Here's the drawing with two shaded views (mm, measured from the low corner). I have some questions. A direction names the side the tool comes from. Coordinates: 2 decimals unless noted, no trailing zeros. Loops run counter-clockwise (first coordinate to the right, second up) from the corner with the lowest first, then second, coordinate; pieces in that order, holes last. Notation, with made-up numbers: (62, -7) - (115, -7) arc R21 ccw to (115, 27) - close; hole circle Ø1 at (-33.5, 47). An arc over 180 degrees is marked (long way). Use a Markdown table: item, result.
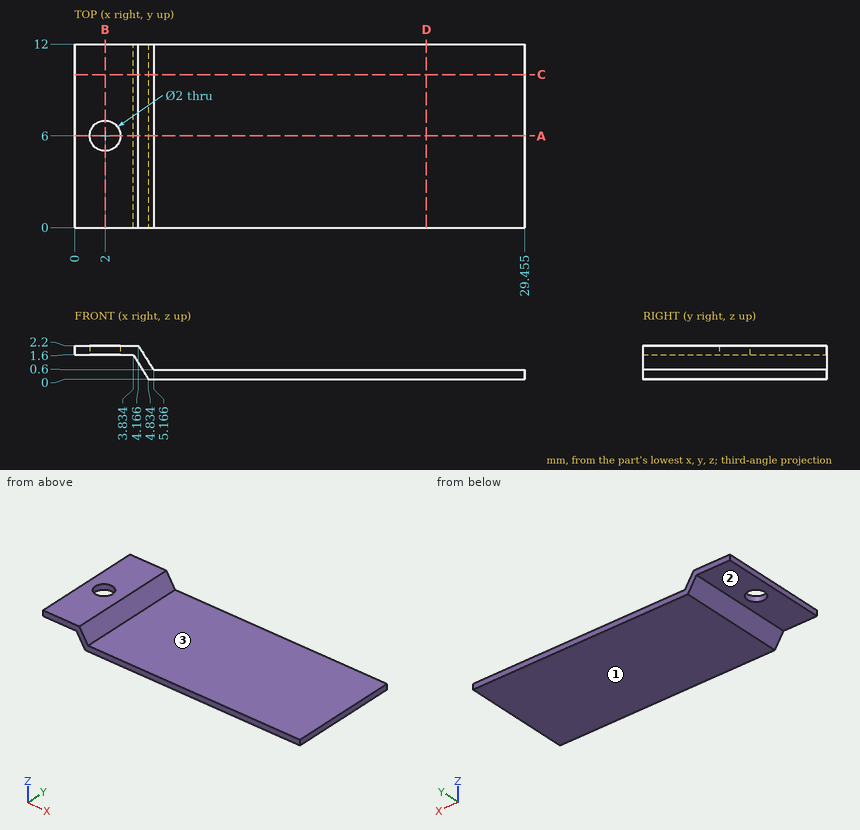
Q1. I want a section at D-D, the plane x = 23. Write out the boundary of the cut face in (y, z).
Check values:
| item | result |
|---|---|
| outline | (0, 0) - (12, 0) - (12, 0.6) - (0, 0.6) - close |
Q2. I want a section at A-A, the plane y = 6. Write out the boundary of the cut face in (x, z) (1 decimal), then the cut area to 3 significant figures.
Check values:
| item | result |
|---|---|
| outline | (0, 1.6) - (1, 1.6) - (1, 2.2) - (0, 2.2) - close; (3, 1.6) - (3.8, 1.6) - (4.8, 0) - (29.5, 0) - (29.5, 0.6) - (5.2, 0.6) - (4.2, 2.2) - (3, 2.2) - close |
| area | 17.0 mm^2 |
Q3. Please list where these lines run through material, in increasing order: L1, parallel to Z at x = 24.5, y = 4.5; L2, parallel to X at y = 6, z = 2.1; L3, parallel to X at y = 5.5, z = 1.7 (1 decimal). Write a range as from..to.
Check values:
| item | result |
|---|---|
| L1 | 0..0.6 |
| L2 | 0..1, 3..4.23 |
| L3 | 0..1.1, 2.9..4.5 |
Q4. I want a section at B-B, the plane x = 2. Write out the boundary of the cut face in (y, z).
Check values:
| item | result |
|---|---|
| outline | (0, 1.6) - (5, 1.6) - (5, 2.2) - (0, 2.2) - close; (7, 1.6) - (12, 1.6) - (12, 2.2) - (7, 2.2) - close |
Q5. Which directions (+Z, -Z, +X, -X, +Y, -Y) give clear straight access to the entire face, cutting with the end or side of a thin tool? Please do the marked faces 1, 2 and 3.
Check values:
| item | result |
|---|---|
| face 1 | -Z, +X, -X, +Y, -Y |
| face 2 | -Z, -X, +Y, -Y |
| face 3 | +Z, +X, +Y, -Y |
Q6. Will these pins go through, and if not, where does the flat tip stop? P1, Ø1, axis at x = 16.5, y = 8, coming from the +Z side; P2, Ø1.9, axis at x = 3, y = 5, coming from the -Z side (1 decimal); P3, Ø1, axis at y = 1.5, z = 1, coming from the +X side (1 decimal).
Check values:
| item | result |
|---|---|
| P1 | z = 0.6 |
| P2 | z = 1.4 |
| P3 | x = 29.5 |
Q7. I want a section at C-C, the plane y = 10. Write out the boundary of the cut face in (x, z) (1 decimal), then the cut area to 3 significant figures.
Check values:
| item | result |
|---|---|
| outline | (0, 1.6) - (3.8, 1.6) - (4.8, 0) - (29.5, 0) - (29.5, 0.6) - (5.2, 0.6) - (4.2, 2.2) - (0, 2.2) - close |
| area | 18.2 mm^2 |
